from build123d import *

# Parameters (mm, degrees)
F0_W     = 19.05
F0_H     = 63.5
F1_DEPTH = 19.05
F2_R     = 7.9375
F3_DEPTH = 19.05


with BuildPart() as f1:
    # F0 (on Top) → F1 (new body)
    with BuildSketch(Plane.XY):
        Polygon((762, 1371.6), (50.8, 1371.6), (50.8, 299.550803), (279.4, 299.550803), (279.4, 197.950803), (279.4, -5.249197), (533.4, -5.249197), (533.4, 197.950803), (533.4, 299.550803), (762, 299.550803), align=None)
        with Locations((168.275, 1149.35)):
            Rectangle(F0_W, F0_H, mode=Mode.SUBTRACT)
        with Locations((168.275, 1289.05)):
            Rectangle(F0_W, F0_H, mode=Mode.SUBTRACT)
        with Locations((644.525, 1149.35)):
            Rectangle(F0_W, F0_H, mode=Mode.SUBTRACT)
        with Locations((644.525, 1289.05)):
            Rectangle(F0_W, F0_H, mode=Mode.SUBTRACT)
    extrude(amount=F1_DEPTH)

    # F2 (on face) → F3 (cut, through all)
    with BuildSketch(Plane.XY.offset(19.05)):
        with Locations((406.4, 45.550803)):
            Circle(F2_R)
    extrude(amount=-F3_DEPTH, mode=Mode.SUBTRACT)


solid = f1.part
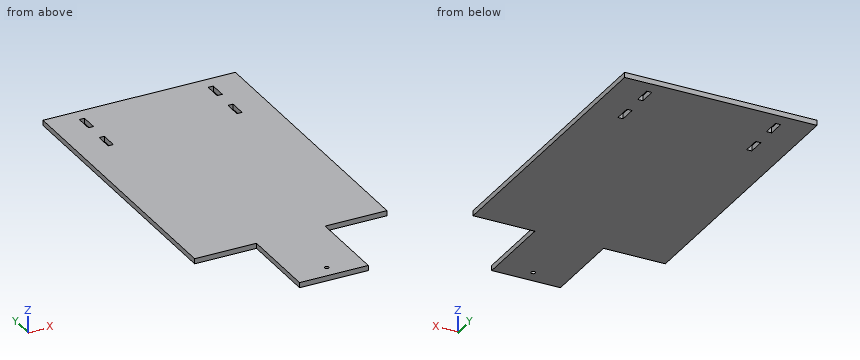
Work out the finished part from the listing and answer in its coordinate system (mm). Give positions to 0.01 mm unless a question says otherwise; leave off trailing zeros. Loops run counter-clockwise (first coordinate to the right, second up) from the corner with the lowest first, then second, coordinate; pieces in that order, holes last. Notation, with made-up numbers: (20.5, -15) -> (55.5, -15) arc R36 cw to (55.5, 24) -> close; hole circle Ø1 at (80.25, 38). An arc over 180 degrees is marked (long way). Use a Markdown table: item, result. Add a question column.
1) Consider line 1 along Y through (x, z) = (406.4, 10.5); line 2 along X through (y, z) = (164.5, 5.25); line 3 along Y through (x, z) = (131.5, 11.75). Determine where each line is inside the solid, lowest interval first.
2) The part is cut by section A-A, the plane z = 15.25. Count the separate pieces of the cut face and the enclosed holes in it, plus the area to 3 significant figures.
3) Each of these flat-tipped pins is pushed along its axis until it touches: P1, Ø5.5, axis at y = 120.5, z = 11.5, coming from the -X side; P2, Ø9.5, axis at x = 646, z = 11, coming from the -Y side. Where does it stop, or does it pass through?
4) The part is cut by section B-B, the plane x = 140. Determine the outline of the cut face in (y, z).
Reported:
| question | item | result |
|---|---|---|
| 1 | line 1 | y = -5.25 to 37.61, 53.49 to 1371.6 |
| 1 | line 2 | x = 279.4 to 533.4 |
| 1 | line 3 | y = 299.55 to 1371.6 |
| 2 | separate pieces | 1 |
| 2 | enclosed holes | 5 |
| 2 | area | 835,000 mm^2 |
| 3 | P1 | stops at x = 279.4 |
| 3 | P2 | stops at y = 299.55 |
| 4 | outline | (299.55, 0) -> (1371.6, 0) -> (1371.6, 19.05) -> (299.55, 19.05) -> close |
